Geometry: final body of the model. Coordinates: model frame, mm. Face numbers are marked on the shaded views. A direction names the side the tool comes from. Round coordinates to 2 decimals unless told otherwise and drop trailing zeros. Order: outer loops, then holes, each group sorted by start corner. A loop starts at its lowest first (then second) coordinate and runs counter-clockwise, first axis right, second up. Notation, with made-up numbers: (52, -7) - (69, -7) arc R23 cw to (69, 14) - close; hole circle Ø5 at (68.5, 29.5). An arc over 180 degrees is marked (long way). Put each result on its own line as item: value. Start each with the question number.
(1) Material intervals for L1, parallel to Y at x = -22.75, z = 24; L2, parallel to Z at x = 71.5, y = -18; L3, parallel to X at y = -8, z = 28.5, sorted ascending. Write a range as [from, to].
(2) Pull-direction query (Y, two-part tool) for the marked faces 3, 4 and 5; classes: released by +Y, released by -Y, zero draft, split by the parting line, or undercut.
(3) Section C-C (z = 28). Output: boundary loops of the cut face in (x, y).
(4) Pin query (flat end, axial travel): P1, Ø10, axis at y = -12, z = 28.5, coming from the +X side; P2, Ø1, axis at x = 151.5, y = 22.5, coming from the +Z side; P3, Ø6, axis at x = 88, z = -0.5, coming from the -Y side; P4, Ø3, axis at x = 92, y = 5, coming from the -Z side. Return the tip coordinate at first contact, or that it passes through.
(5) Section D-D (z = -9). Output: boundary loops of the cut face in (x, y), and give its area (3 significant figures).
(6) Section B-B (x = 147). Output: boundary loops of the cut face in (y, z).
(7) Access query for the marked faces 1 and 2. Directions: +Z, -Z, +X, -X, +Y, -Y. A direction counts if a zero-diameter tool reaches every point of the face in a straight line with its end or side. Return the directions, or none.
(8) Section A-A (y = 0). Count the separate pieces of the cut face and the enclosed holes in it, and give its area (3 significant figures).
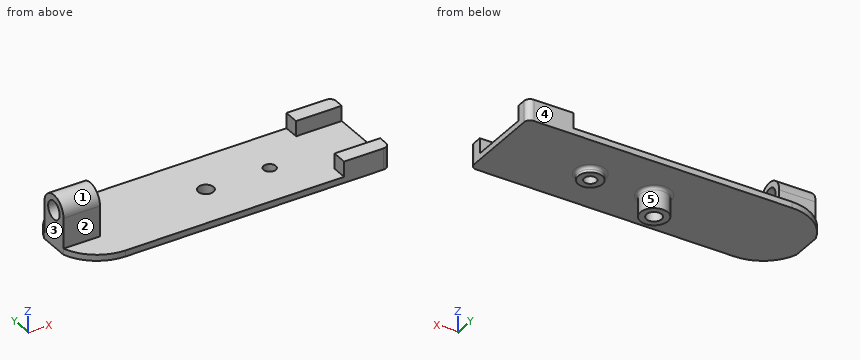
from build123d import *

# Parameters (mm, degrees)
BASE_EXTRUSION_DEPTH    = 4
ESQUISSE2_W             = 30
ESQUISSE2_H             = 10
BOSS_EXTRU_1_DEPTH      = 10
ESQUISSE3_R             = 8
ESQUISSE3_R_2           = 9
BOSS_EXTRU_2_DEPTH      = 4
ESQUISSE4_R             = 4
ENL_V_MAT_EXTRU_1_DEPTH = 178.20370881
ESQUISSE5_R             = 5
ENL_V_MAT_EXTRU_2_DEPTH = 178.20370881
CONG_1_R                = 2
CONG_2_R                = 4
ESQUISSE6_R             = 6
BOSS_EXTRU_3_DEPTH      = 24
ESQUISSE7_R             = 9
ESQUISSE7_R_2           = 5
BOSS_EXTRU_4_DEPTH      = 10


with BuildPart() as part:
    # Esquisse1 → Base-Extrusion (new body)
    with BuildSketch(Plane.XY):
        with BuildLine():
            Line((0, 30), (173.715728753, 30))
            Line((173.715728753, 30), (173.715728753, -30))
            Line((173.715728753, -30), (0, -30))
            ThreePointArc((0, -30), (-17.320508076, -24.494897428), (-28.284271247, -10))
            Line((-28.284271247, -10), (-28.284271247, 10))
            ThreePointArc((-28.284271247, 10), (-17.320508076, 24.494897428), (0, 30))
        make_face()
    extrude(amount=BASE_EXTRUSION_DEPTH)

    # Esquisse2 → Boss.-Extru.1 (add)
    with BuildSketch(Plane.XY.offset(4)):
        with Locations((158.715728753, 25)):
            Rectangle(ESQUISSE2_W, ESQUISSE2_H)
        with Locations((158.715728753, -25)):
            Rectangle(ESQUISSE2_W, ESQUISSE2_H)
    extrude(amount=BOSS_EXTRU_1_DEPTH)

    # Esquisse3 → Boss.-Extru.2 (add)
    with BuildSketch(Plane(origin=(0, 0, 0), x_dir=(-1, 0, 0), z_dir=(0, 0, -1))):
        with Locations(Location((-113.715728753, 0, 0), (0, 0, 180))):
            Circle(ESQUISSE3_R)
        with Locations(Location((-71.715728753, 0, 0), (0, 0, 180))):
            Circle(ESQUISSE3_R_2)
    extrude(amount=BOSS_EXTRU_2_DEPTH)

    # Esquisse4 → Enlèv. mat.-Extru.1 (cut, through all)
    with BuildSketch(Plane(origin=(0, 0, -4), x_dir=(-1, 0, 0), z_dir=(0, 0, -1))):
        with Locations((-113.715728753, 0)):
            Circle(ESQUISSE4_R)
    extrude(amount=-ENL_V_MAT_EXTRU_1_DEPTH, mode=Mode.SUBTRACT)

    # Esquisse5 → Enlèv. mat.-Extru.2 (cut, through all)
    with BuildSketch(Plane(origin=(0, 0, -4), x_dir=(-1, 0, 0), z_dir=(0, 0, -1))):
        with Locations((-71.715728753, 0)):
            Circle(ESQUISSE5_R)
    extrude(amount=-ENL_V_MAT_EXTRU_2_DEPTH, mode=Mode.SUBTRACT)

    # Congé1
    cong_1_edges = [part.edges().sort_by_distance(p)[0] for p in [
        (105.715728753, 0, 0),
        (62.715728753, 0, 0),
    ]]
    fillet(cong_1_edges, radius=CONG_1_R)

    # Congé2
    cong_2_edges = [part.edges().sort_by_distance(p)[0] for p in [
        (173.715728753, 30, 7),
        (173.715728753, -30, 7),
    ]]
    fillet(cong_2_edges, radius=CONG_2_R)

    # Esquisse6 → Boss.-Extru.3 (add)
    with BuildSketch(Plane.ZY.offset(28.284271247)):
        with BuildLine():
            Line((0, 10), (24, 10))
            ThreePointArc((24, 10), (34, 0), (24, -10))
            Line((24, -10), (0, -10))
            Line((0, -10), (0, 10))
        make_face()
        with Locations((24, 0)):
            Circle(ESQUISSE6_R, mode=Mode.SUBTRACT)
    extrude(amount=-BOSS_EXTRU_3_DEPTH)

    # Esquisse7 → Boss.-Extru.4 (add)
    with BuildSketch(Plane(origin=(0, 0, -4), x_dir=(-1, 0, 0), z_dir=(0, 0, -1))):
        with Locations(Location((-71.715728753, 0, 0), (0, 0, 180))):
            Circle(ESQUISSE7_R)
        with Locations((-71.715728753, 0)):
            Circle(ESQUISSE7_R_2, mode=Mode.SUBTRACT)
    extrude(amount=BOSS_EXTRU_4_DEPTH)


solid = part.part
Checks:
1. L1: y = [-10, -6], [6, 10]
1. L2: z = [0, 4]
1. L3: x = [-28.28, -4.28]
2. face 3: zero draft
2. face 4: released by +Y
2. face 5: split by the parting line
3. outline: (-28.28, -9.17) - (-4.28, -9.17) - (-4.28, -4.47) - (-28.28, -4.47) - close; (-28.28, 4.47) - (-4.28, 4.47) - (-4.28, 9.17) - (-28.28, 9.17) - close
4. P1: stops at x = -4.28
4. P2: stops at z = 14
4. P3: stops at y = -30
4. P4: stops at z = 0
5. outline: circle Ø18 at (71.72, 0); hole circle Ø10 at (71.72, 0)
5. area: 176 mm²
6. outline: (-30, 0) - (30, 0) - (30, 14) - (20, 14) - (20, 4) - (-20, 4) - (-20, 14) - (-30, 14) - close
7. face 1: +Z, +X, -X
7. face 2: +Z, +X, -X, -Y
8. separate pieces: 4
8. enclosed holes: 0
8. area: 1,320 mm²
